The drawing under review shows one solid part. Ordinate dimensions are in mm from its lowest x, y, z. Round coordinates to 2 decimals unless told otherwise and drop trailing zeros. Write each loop counter-clockwise with the first axis right and the second up, starting at its lowest first coordinate (ties: lowest second). Pieces come first, ordered by that corner, then holes. Notation, with made-up numbers: (14.5, 80) -> (28.5, 80) arc R16 ccw to (28.5, 88) -> close; hole circle Ø2 at (-8.75, 56). An arc over 180 degrees is marked (long way). Answer in a Markdown table with one row per item.
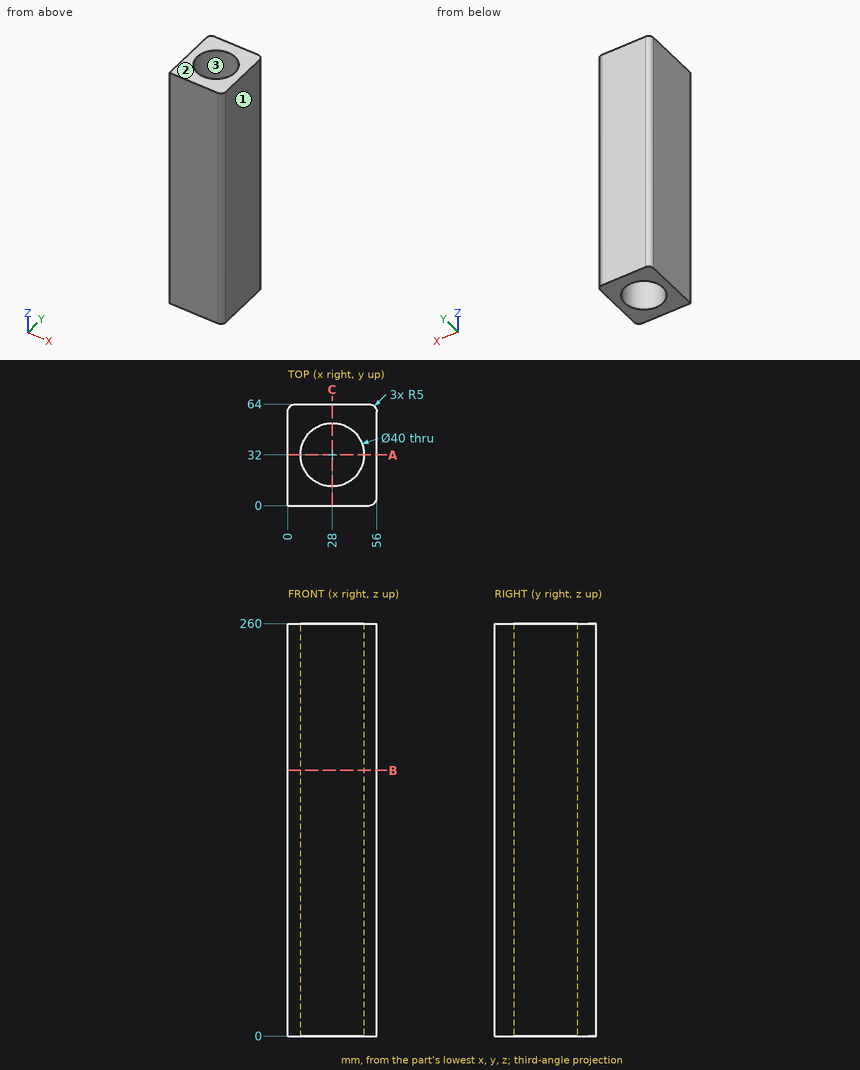
1) Clearance check with a flat-ended pin moving along its axis: pin 1 Ø12 at (y, z) = (31.5, 31) entering from -X. State where the tip first meets the part, or that it passes through.
Solved:
| item | result |
|---|---|
| pin 1 | x = 0 |
2) Consider section A-A on y = 32. State the section outline as (x, z) points.
Solved:
| item | result |
|---|---|
| outline | (0, 0) -> (8, 0) -> (8, 260) -> (0, 260) -> close; (48, 0) -> (56, 0) -> (56, 260) -> (48, 260) -> close |
3) For line 1 (Y direction, x = 28, z = 197); line 2 (Y direction, x = 17.5, z = 71); line 3 (X direction, y = 36, z = 248), list the stretches that pass through material, from the lowest coordinate up. Write a range as [from, to].
Solved:
| item | result |
|---|---|
| line 1 | [0, 12], [52, 64] |
| line 2 | [0, 14.98], [49.02, 64] |
| line 3 | [0, 8.4], [47.6, 56] |
4) Consider section B-B on z = 167.5. State the section outline as (x, y) points.
Solved:
| item | result |
|---|---|
| outline | (0, 0) -> (51, 0) arc R5 ccw to (56, 5) -> (56, 59) arc R5 ccw to (51, 64) -> (5, 64) arc R5 ccw to (0, 59) -> close; hole circle Ø40 at (28, 32) |
5) Mouldability with a two-part tool opening along X and no side actions: class the marked faces 1, 2 and 3 as pulls with the +X half, pulls with the -X half, needs draft (parallel to the pull), parting line crosses it, or undercut.
Solved:
| item | result |
|---|---|
| face 1 | pulls with the +X half |
| face 2 | needs draft |
| face 3 | undercut |
6) Consider section C-C on x = 28. State the section outline as (y, z) points.
Solved:
| item | result |
|---|---|
| outline | (0, 0) -> (12, 0) -> (12, 260) -> (0, 260) -> close; (52, 0) -> (64, 0) -> (64, 260) -> (52, 260) -> close |
